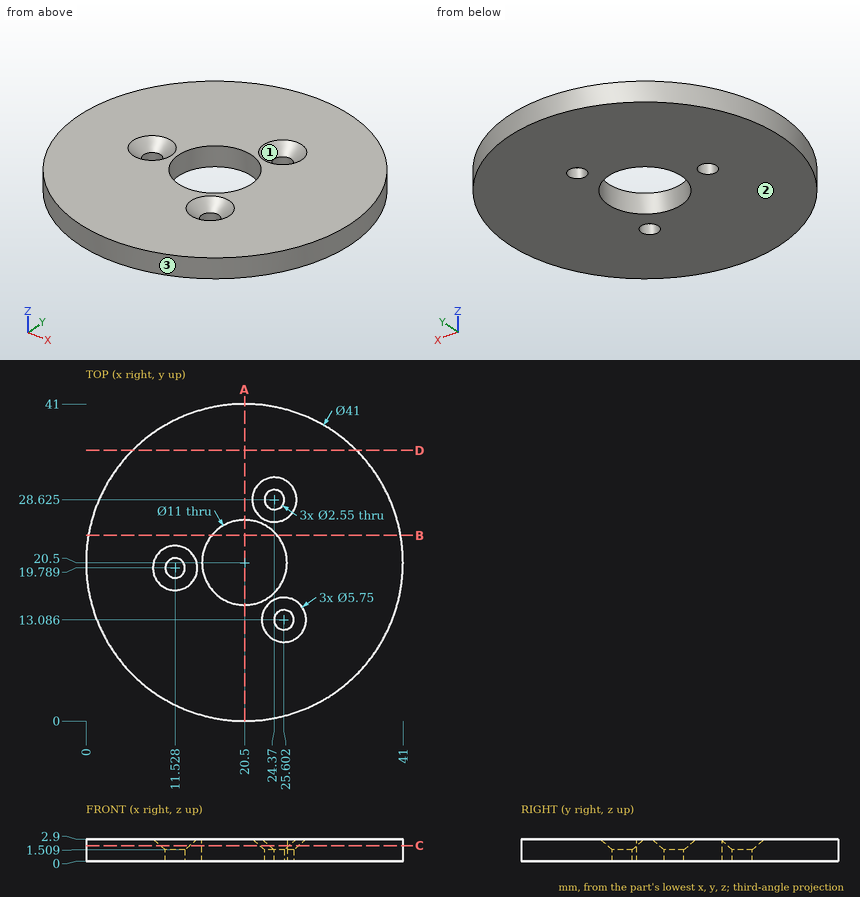
Print and shaded views of the part. All mm, measured from the part's lowest x, y and z. Coordinates: 2 decimals unless noted, no trailing zeros. Write each loop counter-clockwise with the first axis right and the second up, starting at its lowest first coordinate (ties: lowest second). Pieces come first, ordered by that corner, then holes. Notation, with made-up numbers: M 58,47 L 116,47 A23 ccw 116,70 Z; hole C 26,34 d2. An arc over 180 degrees is marked long. Return JSON: item names as keys, results as strings.
1. Saw through at B-B, the plane y = 24. Write the cut outline in (x, z).
Determined:
{"outline": "M 0.3,0 L 16.26,0 L 16.26,2.9 L 0.3,2.9 Z; M 24.74,0 L 40.7,0 L 40.7,2.9 L 24.74,2.9 Z"}
2. Pull direction X, two halves, no side cores. Call the marked faces 1, 2 and 3: pulls with the +X half, pulls with the -X half, needs draft (parallel to the pull), parting line crosses it, or undercut.
Determined:
{"face 1": "undercut", "face 2": "needs draft", "face 3": "parting line crosses it"}
3. Saw through at C-C, the plane z = 2.05. Write the cut outline in (x, y) (1 decimal).
Determined:
{"outline": "C 20.5,20.5 d41; hole C 11.5,19.8 d3.8; hole C 20.5,20.5 d11; hole C 24.4,28.6 d3.8; hole C 25.6,13.1 d3.8"}
4. Saw through at D-D, the plane y = 35. Write the cut outline in (x, z).
Determined:
{"outline": "M 6.01,0 L 34.99,0 L 34.99,2.9 L 6.01,2.9 Z"}
5. Probe L1, parallel to Y at x = 20.5, z = 2.15; L2, parallel to X at y = 21.5, z = 0.9 (1 decimal). List the from-to ranges inside material, lowest first.
Determined:
{"L1": "0 to 15, 26 to 41", "L2": "0 to 15.1, 25.9 to 41"}
6. Saw through at A-A, the plane x = 20.5. Write the cut outline in (y, z).
Determined:
{"outline": "M 0,0 L 15,0 L 15,2.9 L 0,2.9 Z; M 26,0 L 41,0 L 41,2.9 L 26,2.9 Z"}
7. Flat gauge pins, fed straight in: pin 1 Ø3 at (x, y) = (11.53, 19.79) entering from -Z; pin 2 Ø1.5 at (x, z) = (7.5, 1.5) entering from +Y; pin 3 Ø1.5 at (x, z) = (5, 2) entering from +Y; pin 4 Ø1.5 at (x, z) = (7, 2.5) entering from +Y. Where does each tip first touch, or does it go through?
Determined:
{"pin 1": "z = 0", "pin 2": "y = 36.94", "pin 3": "y = 34.74", "pin 4": "y = 36.55"}
